```python
from build123d import *

# Parameters (mm, degrees)
SKETCH1_W             = 7
SKETCH1_H             = 3
BOSS_EXTRUDE1_DEPTH   = 3
F_4_CLEARANCE_HOLE1_D = 3.2639


with BuildPart() as part:
    # Sketch1 → Boss-Extrude1 (new body)
    with BuildSketch(Plane(origin=(0, 0, 0), x_dir=(1, 0, 0), z_dir=(0, 1, 0))):
        with Locations((3.5, 1.5)):
            Rectangle(SKETCH1_W, SKETCH1_H)
        with BuildLine():
            Line((-2.5, 3), (0, 3))
            Line((0, 3), (7, 3))
            Line((7, 3), (17, 3))
            Line((17, 3), (24, 3))
            Line((24, 3), (26.5, 3))
            Line((26.5, 3), (26.5, 9))
            ThreePointArc((26.5, 9), (24.742640687, 13.242640687), (20.5, 15))
            Line((20.5, 15), (3.5, 15))
            ThreePointArc((3.5, 15), (-0.742640687, 13.242640687), (-2.5, 9))
            Line((-2.5, 9), (-2.5, 3))
        make_face()
        with Locations((20.5, 1.5)):
            Rectangle(SKETCH1_W, SKETCH1_H)
    extrude(amount=BOSS_EXTRUDE1_DEPTH)

    # #4 Clearance Hole1 (through all)
    with Locations(Plane(origin=(0, 3, 0), x_dir=(1, 0, 0), z_dir=(0, 1, 0))):
        with Locations((3.5, 9), (20.5, 9)):
            Hole(F_4_CLEARANCE_HOLE1_D / 2)


solid = part.part
```
Build history of the part. All positions in model axes, mm. A direction names the side the tool comes from. Give positions to 0.01 mm unless a question says otherwise; leave off trailing zeros. Order: outer loops, then holes, each group sorted by start corner. A loop starts at its lowest first (then second) coordinate and runs counter-clockwise, first axis right, second up. Notation, with made-up numbers: M 88,10 L 130,10 A20 ccw 130,18 Z; hole C 32,15 d10. An arc over 180 degrees is marked long. Return JSON: item names as keys, results as strings.
Q1. Band-saw the part on A-A (y = 2.6). Give the cut face in (x, z), then the cut area to 3 significant figures.
Answer list:
{"outline": "M -2.5,-9 A6 ccw 3.5,-15 L 20.5,-15 A6 ccw 26.5,-9 L 26.5,-3 L 24,-3 L 24,0 L 17,0 L 17,-3 L 7,-3 L 7,0 L 0,0 L 0,-3 L -2.5,-3 Z; hole C 3.5,-9 d3.26; hole C 20.5,-9 d3.26", "area": "358 mm^2"}
Q2. Band-saw the part on B-B (x = 21.75). Give the cut face in (y, z).
Answer list:
{"outline": "M 0,-14.87 L 3,-14.87 L 3,-10.05 L 0,-10.05 Z; M 0,-7.95 L 3,-7.95 L 3,0 L 0,0 Z"}
Q3. Band-saw the part on D-D (z = -12.75). Give the cut face in (x, y).
Answer list:
{"outline": "M -1.18,0 L 25.18,0 L 25.18,3 L -1.18,3 Z"}
Q4. Flat gauge pins, fed straight in: pin 1 (0.9 mm diameter, centred on y = 1, z = -1, fed in from +X); pin 2 (0.8 mm diameter, centred on x = 25, y = 2, fed in from +Z); pin 3 (1.5 mm diameter, centred on y = 1.5, z = -2, fed in from -X); pin 4 (4 mm diameter, centred on x = 20.5, z = -9, fed in from +Y). Where does each tip first touch, or does it go through?
Answer list:
{"pin 1": "stops at x = 24", "pin 2": "stops at z = -3", "pin 3": "stops at x = 0", "pin 4": "stops at y = 3"}
Q5. 3-axis set-ups, long thin cutter, end or side, ignore diameter. For faces 4 (the face through (0, 1, -1)), 5 (the face through (26.5, 1, -6)), 6 (the face through (25, 1, -3)), 7 (the face through (17, 1, -1)): which of +Z, -Z, +X, -X, +Y, -Y reach the whole face in a straight line?
Answer list:
{"face 4": "+Z, -X, +Y, -Y", "face 5": "+Z, -Z, +X, +Y, -Y", "face 6": "+Z, +X, +Y, -Y", "face 7": "+Z, +Y, -Y"}
Q6. Wall check: probe 1 along X at (y, z) = (1.5, -9); probe 2 along Z at (x, y) = (3.5, 2); probe 3 along X at (y, z) = (1.1, -10). Give the ranges that are in metal, low to high. Write a range as from..to.
Answer list:
{"probe 1": "x = -2.5..1.87, 5.13..18.87, 22.13..26.5", "probe 2": "z = -15..-10.63, -7.37..0", "probe 3": "x = -2.42..2.21, 4.79..19.21, 21.79..26.42"}
Q7. Two-plate mould, pull along Z, no slides. Class faces 1 (the face through (3.854, 1.479, -7.407)), 2 (the face through (12, 1, -15)), 3 (the face through (12, 1, -3)): pulls with the +Z half, pulls with the -Z half, needs draft (parallel to the pull), parting line crosses it, or undercut.
Answer list:
{"face 1": "undercut", "face 2": "pulls with the -Z half", "face 3": "pulls with the +Z half"}
Q8. Band-saw the part on C-C (x = 15.25). Give the cut face in (y, z), then the cut area to 3 significant figures.
Answer list:
{"outline": "M 0,-15 L 3,-15 L 3,-3 L 0,-3 Z", "area": "36.0 mm^2"}
